Work out the finished part from the listing and answer in its coordinate system (mm). Face numbers are marked on the shaded views. Round coordinates to 2 decimals unless told otherwise and drop trailing zeros. Order: outer loops, then holes, each group sorted by start corner. A loop starts at its lowest first (then second) coordinate and runs counter-clockwise, first axis right, second up. Notation, with made-up numbers: (-10.5, -15.75) - (26.5, -15.75) arc R21 ccw to (26.5, -3.75) - close; hole circle Ø3 at (-21, -15.75). An arc over 180 degrees is marked (long way). Use one line per item in the form item = value. Start each with the question number.
Q1. For a pull along Y with two mould halves and no side action, classify the marked faces 1, 2 and 3 as +Y half, -Y half, draft (parallel to the pull), parting line (faces both ways), or undercut.
Q2. Find the intervals of material crossed by line 1 (Y direction, x = 0, z = 3.5); line 2 (X direction, y = 0.5, z = 10.5); line 3 (Y direction, x = 0, z = 10), in increasing order. Write a range as [from, to].
Q3. The part is cut by section C-C on z = 8. Determine the outline of the cut face in (x, y).
Q4. The part is cut by section D-D on y = -13. Determine the outline of the cut face in (x, z), plus the area to 3 significant figures.
Q5. Given P1, Ø2, axis at x = 0, z = 8, coming from the -Y side; P2, Ø6, axis at y = -3, z = 11, coming from the +X side; P3, Ø5, axis at x = 11.5, y = 5.5, coming from the +Z side; P4, Ø8, axis at x = 10.5, z = 4, coming from the +Y side, each flat-ended and moving along its own axis, determine where each tip first touches the part or whether it passes through.
Q6. The part is cut by section A-A on y = 0. Determine the outline of the cut face in (x, z).
from build123d import *

# Parameters (mm, degrees)
ESQUISSE1_R             = 20
BOSS_EXTRU_1_DEPTH      = 16
ESQUISSE2_R             = 20
ESQUISSE2_R_2           = 12
ENL_V_MAT_EXTRU_1_DEPTH = 12
ESQUISSE3_R             = 11
ENL_V_MAT_EXTRU_2_DEPTH = 17


with BuildPart() as part:
    # Esquisse1 → Boss.-Extru.1 (new body)
    with BuildSketch(Plane.XY):
        Circle(ESQUISSE1_R)
    extrude(amount=BOSS_EXTRU_1_DEPTH)

    # Esquisse2 → Enlèv. mat.-Extru.1 (cut)
    with BuildSketch(Plane.XY.offset(16)):
        Circle(ESQUISSE2_R)
        Circle(ESQUISSE2_R_2, mode=Mode.SUBTRACT)
    extrude(amount=-ENL_V_MAT_EXTRU_1_DEPTH, mode=Mode.SUBTRACT)

    # Esquisse3 → Enlèv. mat.-Extru.2 (cut, through all)
    with BuildSketch(Plane.XY.offset(16)):
        Circle(ESQUISSE3_R)
    extrude(amount=-ENL_V_MAT_EXTRU_2_DEPTH, mode=Mode.SUBTRACT)


solid = part.part
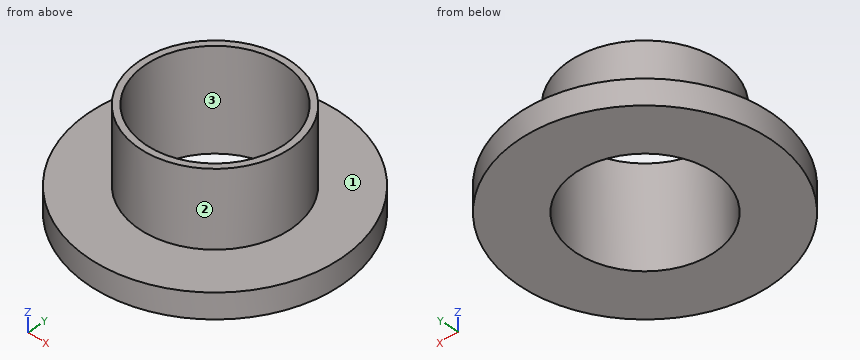
Found:
q1.face_1 = draft
q1.face_2 = parting line
q1.face_3 = undercut
q2.line_1 = [-20, -11], [11, 20]
q2.line_2 = [-11.99, -10.99], [10.99, 11.99]
q2.line_3 = [-12, -11], [11, 12]
q3.outline = circle Ø24 at (0, 0); hole circle Ø22 at (0, 0)
q4.outline = (-15.2, 0) - (15.2, 0) - (15.2, 4) - (-15.2, 4) - close
q4.area = 122 mm²
q5.P1 = -12
q5.P2 = 12
q5.P3 = 16
q5.P4 = 18.91
q6.outline = (-20, 0) - (-11, 0) - (-11, 16) - (-12, 16) - (-12, 4) - (-20, 4) - close; (11, 0) - (20, 0) - (20, 4) - (12, 4) - (12, 16) - (11, 16) - close
